The model under review builds one solid part; all positions refer to its coordinate system, in mm. A direction names the side the tool comes from. Round coordinates to 2 decimals unless told otherwise and drop trailing zeros. Write each loop counter-clockwise with the first axis right and the second up, starting at its lowest first coordinate (ties: lowest second). Pieces come first, ordered by that corner, then holes. Notation, with made-up numbers: M -7,85 L 18,85 A18 ccw 18,114 Z; hole C 81,-16 d6. An arc over 180 degrees is marked long. One line per item, written item: value. Start each with the question number.
1) Take a section at D-D, the plane x = 5.25. Write out the cut boundary in (y, z), and give its area (3 significant figures).
2) Take a section at C-C, the plane y = 5. Write out the cut boundary in (x, z), and give its area (3 significant figures).
3) For P1, Ø4, axis at y = -2, z = -6, coming from the +X side; P2, Ø2, axis at y = -2.5, z = -6.5, coming from the -X side; P3, Ø4, axis at x = -1, z = -6.5, coming from the +Y side, all flat-tipped, find the tip position at first contact; note any pin that passes through.
4) Wall thickness on probe 1 along Y at (x, z) = (0, -6); probe 2 along Z at (x, y) = (-3, -2.25); probe 3 along X at (y, z) = (1, -8.5): over which ranges is each line inside the solid? List them lowest first.
5) Take a section at A-A, the plane x = 0. Write out the cut boundary in (y, z).
6) Tool access review of faces 1 (the face through (-1.3, 1.3, 1.016)), 2 (the face through (2, -3, 0)): name each direction out of +Z, -Z, +X, -X, +Y, -Y from which nothing blocks a thin tool from reaching the whole face with its end or side.
from build123d import *

# Parameters (mm, degrees)
SKETCH1_R        = 3.6322
BASEPULLEY_DEPTH = 8.89
GROOVE_DEPTH     = 4.445
GROOVES_COUNT    = 12
GROOVES_ANGLE    = 330
SKETCH4_W        = 1.016
SKETCH4_H        = 6.35
BORSKE_R         = 1.5875
BORE_DEPTH       = 14.370633343


with BuildPart() as part:
    # Sketch1 → BasePulley (new body)
    with BuildSketch(Plane.XY):
        Circle(SKETCH1_R)
    extrude(amount=-BASEPULLEY_DEPTH)

    # Sketch3 → Groove (cut, symmetric)
    with BuildSketch(Plane.XY.offset(-4.445)):
        with BuildLine():
            Line((-0.5715, 3.6322), (-0.5715, 29.0322))
            Line((-0.5715, 29.0322), (0.5715, 29.0322))
            Line((0.5715, 29.0322), (0.5715, 3.6322))
            Line((0.5715, 3.6322), (0.417017726, 3.207763442))
            ThreePointArc((0.417017726, 3.207763442), (0.370520971, 3.14716769), (0.297676764, 3.1242))
            Line((0.297676764, 3.1242), (-0.297676764, 3.1242))
            ThreePointArc((-0.297676764, 3.1242), (-0.370520971, 3.14716769), (-0.417017726, 3.207763442))
            Line((-0.417017726, 3.207763442), (-0.5715, 3.6322))
        make_face()
    groove = extrude(amount=GROOVE_DEPTH, both=True, mode=Mode.SUBTRACT)

    # Grooves: Groove ×12 about axis
    grooves_axis = Axis((0, 0, -8.89), (0, 0, 1))
    for i in range(1, GROOVES_COUNT):
        add(groove.rotate(grooves_axis, i * GROOVES_ANGLE / (GROOVES_COUNT - 1)), mode=Mode.SUBTRACT)

    # Sketch4 → BaseHub (revolve)
    with BuildSketch(Plane(origin=(0, 0, 0), x_dir=(0, 0, -1), z_dir=(1, 0, 0)), mode=Mode.PRIVATE) as basehub_sk:
        with Locations((-0.508, 3.175)):
            Rectangle(SKETCH4_W, SKETCH4_H)
    revolve(basehub_sk.sketch.rotate(Axis((0, 0, 0), (0, 0, -1)), 90), axis=Axis((0, 0, 0), (0, 0, -1)))

    # BorSke → Bore (cut, through all)
    with BuildSketch(Plane.XY.offset(1.016)):
        Circle(BORSKE_R)
    extrude(amount=-BORE_DEPTH, mode=Mode.SUBTRACT)


solid = part.part
Checked values:
1. outline: M -3.57,0 L 3.57,0 L 3.57,1.02 L -3.57,1.02 Z
1. area: 7.26 mm2
2. outline: M -3.91,0 L 3.91,0 L 3.91,1.02 L -3.91,1.02 Z
2. area: 7.95 mm2
3. P1: stops at x = 3.59
3. P2: stops at x = -2.83
3. P3: stops at y = 3.59
4. probe 1: y = -3.12 to -1.59, 1.59 to 3.12
4. probe 2: z = 0 to 1.02
4. probe 3: x = -3.49 to -1.23, 1.23 to 3.49
5. outline: M -6.35,0 L -3.12,0 L -3.12,-8.89 L -1.59,-8.89 L -1.59,1.02 L -6.35,1.02 Z; M 1.59,-8.89 L 3.12,-8.89 L 3.12,0 L 6.35,0 L 6.35,1.02 L 1.59,1.02 Z
6. face 1: +Z, +X, -X, +Y, -Y
6. face 2: -Z
